Geometry check sheet. Reference: the model listing, model coordinates, mm. A direction names the side the tool comes from. Coordinates: 2 decimals unless noted, no trailing zeros. Write each loop counter-clockwise with the first axis right and the second up, starting at its lowest first coordinate (ties: lowest second). Pieces come first, ordered by that corner, then holes. Notation, with made-up numbers: (-33, 73.5) -> (17, 73.5) arc R17 ccw to (17, 105.5) -> close; hole circle Ø11 at (68, -7.5). An arc over 180 degrees is marked (long way). Put each result on its own line as item: value. Start each with the question number.
from build123d import *

# Parameters (mm, degrees)
CROQUIS1_R              = 13
SALIENTE_EXTRUIR1_DEPTH = 4
CORTAR_EXTRUIR1_DEPTH   = 2


with BuildPart() as part:
    # Croquis1 → Saliente-Extruir1 (new body)
    with BuildSketch(Plane(origin=(0, 0, 0), x_dir=(1, 0, 0), z_dir=(0, 1, 0))):
        with Locations(Location((0, 0, 0), (0, 0, 270))):
            Circle(CROQUIS1_R)
    extrude(amount=SALIENTE_EXTRUIR1_DEPTH)

    # Croquis4 → Cortar-Extruir1 (cut)
    with BuildSketch(Plane(origin=(0, 4, 0), x_dir=(1, 0, 0), z_dir=(0, 1, 0))):
        with BuildLine():
            Line((-3.184010772, -2.387150019), (0.656665628, -15.151411134))
            ThreePointArc((0.656665628, -15.151411134), (3.567700163, -16.877026265), (5.531329778, -14.120936937))
            Line((5.531329778, -14.120936937), (3.877699322, -0.894347681))
            ThreePointArc((3.877699322, -0.894347681), (3.756105044, -0.063772705), (3.599765133, 0.76096834))
            ThreePointArc((3.599765133, 0.76096834), (3.408954999, 1.57842259), (3.184010772, 2.387150019))
            Line((3.184010772, 2.387150019), (-0.656665628, 15.151411134))
            ThreePointArc((-0.656665628, 15.151411134), (-3.567700163, 16.877026265), (-5.531329778, 14.120936937))
            Line((-5.531329778, 14.120936937), (-3.877699322, 0.894347681))
            ThreePointArc((-3.877699322, 0.894347681), (-3.756105044, 0.063772705), (-3.599765133, -0.76096834))
            ThreePointArc((-3.599765133, -0.76096834), (-3.408954999, -1.57842259), (-3.184010772, -2.387150019))
        make_face()
    extrude(amount=-CORTAR_EXTRUIR1_DEPTH, mode=Mode.SUBTRACT)


solid = part.part
Item 1: Access from +Z, -Z, +X, -X, +Y, -Y to the whole of each face (thin tool, end or side, straight path). Record for faces 5 (the flat face through (0, 2, 0)), 6 (the flat face through (-6, 4, 0)).
Item 2: Section check A-A, the plane y = 2.9. Enter the section's corners in (x, z).
Item 3: Section check B-B, the plane z = 0. Enter the section's corners in (x, y).
Item 4: Scan lines: line 1 along Y through (x, z) = (4.5, 8); line 2 along X through (y, z) = (3.5, -1.25); line 3 along X through (y, z) = (2.5, 8.75). Record each from-to range of solid material in increasing order. Write a range as [from, to].
Item 5: Section check D-D, the plane y = 0.75. Enter the section's corners in (x, z).
Item 6: Mould release check, pull along X, two halves, no side actions. Record for faces 1 (the flat face through (7, 4, -1)), 2 (the cylindrical face through (-7.91, 1.972, -10.316)), 3 (the flat face through (4.575, 3.014, 6.47)), 4 (the flat face through (-4.575, 3.014, -6.47)): released by +X, released by -X, zero draft, split by the parting line, or undercut.
Item 7: Section check C-C, the plane x = -2. Enter the section's corners in (y, z), and give its area (3 significant figures).
Item 8: Go/stop test with flat-tipped pins: P1, Ø2, axis at x = -2.5, y = 2, coming from the -Z side; P2, Ø1.5, axis at x = -6, y = 1, coming from the -Z side; P3, Ø10, axis at x = 0.5, z = -2.5, coming from the +Y side; P4, Ø1, axis at x = 8, y = 0.5, coming from the +Z side. Record where each tip stops, or that it passes through.
From the geometry:
1. face 5: +Y
1. face 6: +Z, -Z, +X, -X, +Y
2. outline: (-5.25, -11.89) -> (-3.88, -0.89) arc R20 cw to (-3.18, 2.39) -> (0.01, 13) arc R13 ccw to start; (-0.01, -13) arc R13 ccw to (5.25, 11.89) -> (3.88, 0.89) arc R20 cw to (3.18, -2.39) -> close
3. outline: (-13, 0) -> (13, 0) -> (13, 4) -> (3.75, 4) -> (3.75, 2) -> (-3.75, 2) -> (-3.75, 4) -> (-13, 4) -> close
4. line 1: [0, 2]
4. line 2: [-12.94, -3.92], [3.49, 12.94]
4. line 3: [-9.61, -1.27], [4.86, 9.61]
5. outline: circle Ø26 at (0, 0)
6. face 1: zero draft
6. face 2: split by the parting line
6. face 3: undercut
6. face 4: undercut
7. outline: (0, -12.85) -> (2, -12.85) -> (2, 6.32) -> (4, 6.32) -> (4, 12.85) -> (0, 12.85) -> close
7. area: 64.4 mm²
8. P1: z = -12.91
8. P2: z = -11.89
8. P3: y = 4
8. P4: z = 10.62
